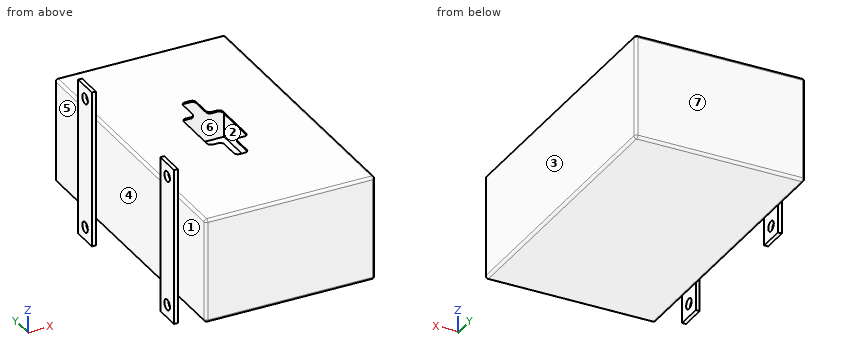
```python
from build123d import *

# Parameters (mm, degrees)
F0_W     = 130
F0_H     = 220
F1_DEPTH = 40
F2_T     = -1
F4_DEPTH = 1
F5_R     = 2
F6_W     = 20
F6_H     = 120
F6_R     = 4
F7_DEPTH = 3


with BuildPart() as f1:
    # F0 (on Top) → F1 (new body, symmetric)
    with BuildSketch(Plane.XY):
        Rectangle(F0_W, F0_H)
    extrude(amount=F1_DEPTH, both=True)

    # F2 (hollow: no face is removed)
    offset(amount=F2_T, mode=Mode.SUBTRACT)

    # F3 (on face) → F4 (cut, through all)
    with BuildSketch(Plane.XY.offset(40)):
        with BuildLine():
            Line((2, 40), (-2, 40))
            ThreePointArc((-2, 40), (-4.1213203436, 39.1213203436), (-5, 37))
            Line((-5, 37), (-5, 23))
            ThreePointArc((-5, 23), (-5.8786796564, 20.8786796564), (-8, 20))
            Line((-8, 20), (-12, 20))
            ThreePointArc((-12, 20), (-14.1213203436, 19.1213203436), (-15, 17))
            Line((-15, 17), (-15, -17))
            ThreePointArc((-15, -17), (-14.1213203436, -19.1213203436), (-12, -20))
            Line((-12, -20), (-8, -20))
            ThreePointArc((-8, -20), (-5.8786796564, -20.8786796564), (-5, -23))
            Line((-5, -23), (-5, -37))
            ThreePointArc((-5, -37), (-4.1213203436, -39.1213203436), (-2, -40))
            Line((-2, -40), (2, -40))
            ThreePointArc((2, -40), (4.1213203436, -39.1213203436), (5, -37))
            Line((5, -37), (5, -23))
            ThreePointArc((5, -23), (5.8786796564, -20.8786796564), (8, -20))
            Line((8, -20), (12, -20))
            ThreePointArc((12, -20), (14.1213203436, -19.1213203436), (15, -17))
            Line((15, -17), (15, 17))
            ThreePointArc((15, 17), (14.1213203436, 19.1213203436), (12, 20))
            Line((12, 20), (8, 20))
            ThreePointArc((8, 20), (5.8786796564, 20.8786796564), (5, 23))
            Line((5, 23), (5, 37))
            ThreePointArc((5, 37), (4.1213203436, 39.1213203436), (2, 40))
        make_face()
    extrude(amount=-F4_DEPTH, mode=Mode.SUBTRACT)

    # F5
    f5_edges = [f1.edges().sort_by_distance(p)[0] for p in [
        (65, 0, -40),
        (65, 110, 0),
        (65, 0, 40),
        (65, -110, 0),
        (-65, 110, 0),
        (-65, 0, -40),
        (-65, -110, 0),
        (-65, 0, 40),
        (0, 110, -40),
        (0, -110, -40),
        (0, 110, 40),
        (0, -110, 40),
    ]]
    fillet(f5_edges, radius=F5_R)

    # F6 (on face) → F7 (join)
    with BuildSketch(Plane(origin=(-65, 0, 0), x_dir=(0, -1, 0), z_dir=(-1, 0, 0))):
        with Locations((-60, 0)):
            Rectangle(F6_W, F6_H)
        with Locations((-60, -50)):
            Circle(F6_R, mode=Mode.SUBTRACT)
        with Locations((-60, 50)):
            Circle(F6_R, mode=Mode.SUBTRACT)
        with Locations((60, 0)):
            Rectangle(F6_W, F6_H)
        with Locations((60, -50)):
            Circle(F6_R, mode=Mode.SUBTRACT)
        with Locations((60, 50)):
            Circle(F6_R, mode=Mode.SUBTRACT)
    extrude(amount=F7_DEPTH)


solid = f1.part
```
Here's how the part is built. I have some questions about the finished solid (model axes, mm). Face numbers are marked on the shaded views. A direction names the side the tool comes from. Coordinates: 2 decimals unless noted, no trailing zeros. Order: outer loops, then holes, each group sorted by start corner. A loop starts at its lowest first (then second) coordinate and runs counter-clockwise, first axis right, second up. Notation, with made-up numbers: M 61,39 L 84,39 A20 cw 84,73 Z; hole C 6.25,-31 d11. An arc over 180 degrees is marked long. Answer as a JSON object with one key per item and string values. Group by question number.
(1) Suppose I cut it at A-A, the plane y = -60. Please give me the cut outline in (x, z), then the cut area to 3 significant figures.
(2) Suppose I cut it at C-C, the plane x = 36. Please give me the cut outline in (y, z).
(3) Suppose I cut it at D-D, the plane z = 50. Please give me the cut outline in (x, y).
(4) For pin 1 (6.5 mm diameter, centred on y = 60, z = 50, fed in from -X); pin 2 (9 mm diameter, centred on y = 60, z = -50, fed in from -X); pin 3 (1 mm diameter, centred on x = -18.5, y = -61.5, fed in from +Z); pin 4 (0.5 mm diameter, centred on y = -28, z = 39.5, fed in from +X), each with a flat end and sliding along its axis, tell me the tip position at first contact or that it passes through.
(5) If we mould it in two halves opening along Y, with no side actions, what happens to the marked faces 5, 6 and 7? For each: released by +Y, released by -Y, zero draft, split by the parting line, or undercut.
(6) Which directions (+Z, -Z, +X, -X, +Y, -Y) give clear straight access to the entire face, cutting with the end or side of a thin tool? Please do the marked faces 1, 2, 3 and 4.
(7) Suppose I cut it at B-B, the plane z = 15. Please give me the cut outline in (x, y).
(8) I need wall thicknesses on probe 1 along Z at (x, y) = (-66.85, -60); probe 2 along Y at (x, z) = (-55, 6); probe 3 along X at (y, z) = (93.5, 20.5). Which ranges of each line are inside material? Lowest first, please.
Values found:
{
 "1": {"outline": "M -68,-60 L -65,-60 L -65,-54 L -68,-54 Z; M -68,-46 L -65,-46 L -65,-38 A2 ccw -63,-40 L 63,-40 A2 ccw 65,-38 L 65,38 A2 ccw 63,40 L -63,40 A2 ccw -65,38 L -65,46 L -68,46 Z; M -68,54 L -65,54 L -65,60 L -68,60 Z; hole M -64,-39 L 64,-39 L 64,39 L -64,39 Z", "area": "725 mm^2"},
 "2": {"outline": "M -110,-38 A2 ccw -108,-40 L 108,-40 A2 ccw 110,-38 L 110,38 A2 ccw 108,40 L -108,40 A2 ccw -110,38 Z; hole M -109,-39 L 109,-39 L 109,39 L -109,39 Z"},
 "3": {"outline": "M -68,-70 L -65,-70 L -65,-64 L -68,-64 Z; M -68,-56 L -65,-56 L -65,-50 L -68,-50 Z; M -68,50 L -65,50 L -65,56 L -68,56 Z; M -68,64 L -65,64 L -65,70 L -68,70 Z"},
 "4": {"pin 1": "passes through", "pin 2": "stops at x = -68", "pin 3": "stops at z = 40", "pin 4": "stops at x = 64.56"},
 "5": {"face 5": "zero draft", "face 6": "undercut", "face 7": "released by +Y"},
 "6": {"face 1": "+Z, -Z, -X, -Y", "face 2": "none", "face 3": "+Z, -Z, +X, +Y, -Y", "face 4": "+Z, -Z, -X"},
 "7": {"outline": "M -68,-70 L -65,-70 L -65,-108 A2 ccw -63,-110 L 63,-110 A2 ccw 65,-108 L 65,108 A2 ccw 63,110 L -63,110 A2 ccw -65,108 L -65,70 L -68,70 L -68,50 L -65,50 L -65,-50 L -68,-50 Z; hole M -64,-109 L 64,-109 L 64,109 L -64,109 Z"},
 "8": {"probe 1": "z = -60 to -54, -46 to 46, 54 to 60", "probe 2": "y = -110 to -109, 109 to 110", "probe 3": "x = -65 to -64, 64 to 65"}
}
